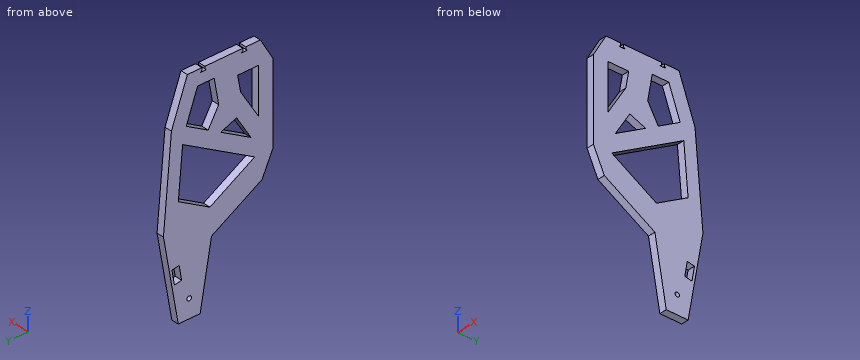
from build123d import *

# Parameters (mm, degrees)
ESQUISSE1_W                  = 300
ESQUISSE1_H                  = 150
BOSS_EXTRU_1_DEPTH           = 5
ESQUISSE2_OUTSIDE_W          = 369.112
ESQUISSE2_OUTSIDE_H          = 219.112
ENL_V_MAT_EXTRU_1_DEPTH      = 5
ENL_V_MAT_EXTRU_2_DEPTH      = 336.559234711
ENL_V_MAT_EXTRU_2_DEPTH_BACK = 336.559234711
ENL_V_MAT_EXTRU_3_DEPTH      = 336.559234711
ENL_V_MAT_EXTRU_3_DEPTH_BACK = 336.559234711
ENL_V_MAT_EXTRU_4_DEPTH      = 336.559234711
ENL_V_MAT_EXTRU_4_DEPTH_BACK = 336.559234711
ESQUISSE5_R                  = 3
ENL_V_MAT_EXTRU_5_DEPTH      = 49


with BuildPart() as part:
    # Esquisse1 → Boss.-Extru.1 (new, symmetric)
    with BuildSketch(Plane(origin=(0, 0, 0), x_dir=(0, 0, -1), z_dir=(1, 0, 0))):
        with Locations((150, 75)):
            Rectangle(ESQUISSE1_W, ESQUISSE1_H)
    extrude(amount=BOSS_EXTRU_1_DEPTH, both=True)

    # Esquisse2 outside → Enlèv. mat.-Extru.1 (cut, symmetric)
    with BuildSketch(Plane(origin=(0, 0, 0), x_dir=(0, 0, -1), z_dir=(1, 0, 0))):
        with Locations((150, 75)):
            Rectangle(ESQUISSE2_OUTSIDE_W, ESQUISSE2_OUTSIDE_H)
        Polygon((0, 117.225703003), (60, 139.063917059), (185, 150), (300, 129.722397219), (300, 99.722397219), (211.741963761, 84.160124165), (171.741963761, 14.878091862), (139.835792798, 0), (29.835792798, 0), (0, 17.225703003), align=None, mode=Mode.SUBTRACT)
    extrude(amount=ENL_V_MAT_EXTRU_1_DEPTH, both=True, mode=Mode.SUBTRACT)

    # Esquisse3 → Enlèv. mat.-Extru.2 (cut, two sides: drawn at the far end of the back side and taken through both)
    with BuildSketch(Plane(origin=(5, 0, 0), x_dir=(0, 0, -1), z_dir=(1, 0, 0)).offset(-ENL_V_MAT_EXTRU_2_DEPTH_BACK)):
        Polygon((20, 103.221552239), (20, 80.493304508), (55, 74.321860183), (80, 88.755616913), (62.679491924, 118.755616913), align=None)
        Polygon((90, 71.435108837), (113.922571241, 30), (81.508057782, 49.831775443), align=None)
        Polygon((82.886751346, 123.755616913), (139.903333355, 25), (175.32640016, 86.354551467), (150.32640016, 129.655821657), align=None)
        Polygon((91.944969354, 20), (30, 20), (30, 48.267236345), (52.117107943, 44.367393479), align=None)
    extrude(amount=ENL_V_MAT_EXTRU_2_DEPTH + ENL_V_MAT_EXTRU_2_DEPTH_BACK, mode=Mode.SUBTRACT)

    # Esquisse4 → Enlèv. mat.-Extru.3 (cut, two sides: drawn at the far end of the back side and taken through both)
    with BuildSketch(Plane(origin=(5, 0, 0), x_dir=(0, 0, -1), z_dir=(1, 0, 0)).offset(-ENL_V_MAT_EXTRU_3_DEPTH_BACK)):
        Polygon((0, 97.225703003), (3, 97.225703003), (5, 99.225703003), (5, 91.225703003), (3, 93.225703003), (0, 93.225703003), align=None)
        Polygon((3, 41.225703003), (0, 41.225703003), (0, 37.225703003), (3, 37.225703003), (5, 35.225703003), (5, 43.225703003), align=None)
    extrude(amount=ENL_V_MAT_EXTRU_3_DEPTH + ENL_V_MAT_EXTRU_3_DEPTH_BACK, mode=Mode.SUBTRACT)

    # Esquisse5 → Enlèv. mat.-Extru.4 (cut, two sides: drawn at the far end of the back side and taken through both)
    with BuildSketch(Plane.ZY.offset(5).offset(-ENL_V_MAT_EXTRU_4_DEPTH_BACK)):
        with Locations((-275, 114.722397219)):
            Circle(ESQUISSE5_R)
    extrude(amount=ENL_V_MAT_EXTRU_4_DEPTH + ENL_V_MAT_EXTRU_4_DEPTH_BACK, mode=Mode.SUBTRACT)

    # Esquisse6 → Enlèv. mat.-Extru.5 (cut)
    with BuildSketch(Plane(origin=(5, 0, 0), x_dir=(0, 0, -1), z_dir=(1, 0, 0))):
        Polygon((230.447006258, 138.381702132), (250.143161319, 134.908738579), (248.406679542, 125.060661049), (228.710524482, 128.533624602), align=None)
    extrude(amount=-ENL_V_MAT_EXTRU_5_DEPTH, mode=Mode.SUBTRACT)


solid = part.part
The listing builds one solid part. Answer for the finished solid, in the listing's coordinates (mm). Give positions to 0.01 mm unless a question says otherwise; leave off trailing zeros. Loops run counter-clockwise (first coordinate to the right, second up) from the corner with the lowest first, then second, coordinate; pieces in that order, holes last. Notation, with made-up numbers: (13, -6) - (38, -6) arc R23 cw to (38, 14) - close; hole circle Ø1 at (60.25, -16.5). An arc over 180 degrees is marked (long way). Use one line per item in the form item = value.
1. Section A-A on z = -275 is taken. Give the vertices of the cut face in (x, y).
Calculated:
outline = (-5, 95.31) - (5, 95.31) - (5, 111.72) - (-5, 111.72) - close; (-5, 117.72) - (5, 117.72) - (5, 134.13) - (-5, 134.13) - close
2. Given pin 1 Ø1.5 at (x, z) = (0, -212.5) entering from +Y; pin 2 Ø0.9 at (x, z) = (-1.5, -1.5) entering from +Y; pin 3 Ø3 at (x, z) = (0.5, -163) entering from +Y; pin 4 Ø9.5 at (y, z) = (114.72, -275) entering from -X, each flat-ended and moving along its own axis, determine where each tip first touches the part or whether it passes through.
Calculated:
pin_1 = 145.28
pin_2 = 117.94
pin_3 = 148.21
pin_4 = -5
3. Section B-B on y = 63.5 is taken. Give the vertices of the cut face in (x, z), then the cut area to 3 significant figures.
Calculated:
outline = (-5, -199.81) - (5, -199.81) - (5, -162.13) - (-5, -162.13) - close; (-5, -117.68) - (5, -117.68) - (5, -94.58) - (-5, -94.58) - close; (-5, -86.88) - (5, -86.88) - (5, 0) - (-5, 0) - close
area = 1,480 mm^2
4. Section D-D on z = -179 is taken. Give the vertices of the cut face in (x, y), then the cut area to 3 significant figures.
Calculated:
outline = (-5, 27.45) - (5, 27.45) - (5, 149.48) - (-5, 149.48) - close
area = 1,220 mm^2
5. Section C-C on x = -0.5 is taken. Count the separate pieces of the cut face and the enclosed holes in it, then the cut area to 3 significant figures.
Calculated:
separate_pieces = 1
enclosed_holes = 6
area = 22,700 mm^2
6. Find the intervals of material crossed by line 1 along Z through (x, y) = (-4.5, 40.5); line 2 along Y through (x, z) = (-3.25, -110); line 3 along Y through (x, z) = (2, -275), in increasing order. Write a range as [from, to].
Calculated:
line_1 = [-186.53, -148.85], [-130.95, -107.86], [-96.76, -58.44], [-30, -5]
line_2 = [0, 32.4], [36.79, 76.79], [126.13, 143.44]
line_3 = [95.31, 111.72], [117.72, 134.13]
